Part model, mm, in its own coordinate system. A direction names the side the tool comes from. Coordinates: 2 decimals unless noted, no trailing zeros. Loops run counter-clockwise (first coordinate to the right, second up) from the corner with the lowest first, then second, coordinate; pieces in that order, holes last. Notation, with made-up numbers: (14, 18.5) -> (32, 18.5) arc R19 ccw to (32, 40.5) -> close; hole circle Ø9 at (37.5, 24). An arc over 180 degrees is marked (long way). Use one line per item in the form item = value. Start each with the question number.
(1) 3-axis set-ups, long thin cutter, end or side, ignore diameter. For faces 1 (the flat face through (6.261, -1.821, -8.524)), 2 (the flat face through (6, -2.473, 4)), 3 (the flat face through (6, 2.607, 4)): which of +Z, -Z, +X, -X, +Y, -Y reach the whole face in a straight line?
(2) Band-saw the part on C-C on y = 3.25. Give the cut face in (x, z) (1 decimal), then the cut area to 3 significant figures.
(3) Band-saw the part on D-D on y = -0.75. Give the cut face in (x, z) (1 decimal), then the cut area to 3 significant figures.
(4) Drill centre lines: L1, parallel to Z at x = 8.5, y = -4 (3 decimals); L2, parallel to Y at x = 5, z = 3.75; L3, parallel to Y at x = 10, z = -4. Where is each one in solid material? Low to high. Write a range as [from, to].
(5) Pin check, flat tips, straight feed: P1, Ø3, axis at x = -3, y = 2, coming from the +Z side; P2, Ø0.7, axis at x = -4, z = 4.5, coming from the +Y side; P3, Ø6, axis at x = -7, y = -4.5, coming from the -Z side. Stop position of each tip, or through.
```python
from build123d import *

# Parameters (mm, degrees)
F0_W      = 25.4
F0_H      = 12.7
F3_DEPTH  = 3.175
F3_FACE_W = 25.4
F3_FACE_H = 12.7
F4_DEPTH  = 3.175
F5_W      = 5.08
F5_H      = 2.286
F7_DEPTH  = 12.7
F6_W      = 5.08
F6_H      = 2.286
F8_DEPTH  = 12.7
F9_DEPTH  = 12.7


with BuildPart() as f3:
    # F0 (on Top) → F3 (new body)
    with BuildSketch(Plane.XY):
        Rectangle(F0_W, F0_H)
    extrude(amount=F3_DEPTH)

    # F3_face (on face) → F4 (join)
    with BuildSketch(Plane(origin=(0, 0, 0), x_dir=(1, 0, 0), z_dir=(0, 0, -1))):
        Rectangle(F3_FACE_W, F3_FACE_H)
    extrude(amount=F4_DEPTH)

    # F1 (on Right) + F5 (on Right) → F7 (join)
    with BuildSketch(Plane.YZ):
        Polygon((3.592102, 6.754402), (0, 10.346504), (-3.592102, 6.754402), (0, 3.1623), align=None)
    with BuildSketch(Plane.YZ):
        with Locations((0.06673, 4.330203)):
            Rectangle(F5_W, F5_H)
    extrude(amount=F7_DEPTH)

    # F6 (on Right) + F2 (on Right) → F8 (join)
    with BuildSketch(Plane.YZ):
        with Locations((-0.087894, -4.272406)):
            Rectangle(F6_W, F6_H)
    with BuildSketch(Plane.YZ):
        Polygon((0, -10.345057), (3.592102, -6.752954), (0, -3.160852), (-3.592102, -6.752954), align=None)
    extrude(amount=F8_DEPTH)

    # F7_face (on face) + F8_face (on face) → F9 (join)
    with BuildSketch(Plane(origin=(0, 0.024156, 6.218296), x_dir=(0, 1, 0), z_dir=(-1, 0, 0))):
        Polygon((-0.04906, 3.031093), (-2.497427, 3.031093), (-2.497427, 0.745093), (-2.33506, 0.745093), (-3.616259, -0.536106), (-0.024156, -4.128208), (3.567946, -0.536106), (2.286747, 0.745093), (2.582573, 0.745093), (2.582573, 3.031093), (0.000747, 3.031093), (-0.011456, 3.043296), (-0.036857, 3.043296), align=None)
    with BuildSketch(Plane(origin=(0, -0.031159, -6.212423), x_dir=(0, 1, 0), z_dir=(-1, 0, 0))):
        Polygon((-2.596735, -3.037423), (2.483265, -3.037423), (2.483265, -0.797017), (2.285713, -0.797017), (3.623261, 0.540531), (0.031159, 4.132633), (-3.560944, 0.540531), (-2.223395, -0.797017), (-2.596735, -0.797017), align=None)
    extrude(amount=F9_DEPTH)


solid = f3.part
```
A:
q1.face_1 = -Z, +X, -X, -Y
q1.face_2 = +X, -X, -Y
q1.face_3 = +X, -X, +Y
q2.outline = (-12.7, -7.1) -> (12.7, -7.1) -> (12.7, -6.4) -> (-12.7, -6.4) -> close; (-12.7, -3.2) -> (12.7, -3.2) -> (12.7, 3.2) -> (-12.7, 3.2) -> close; (-12.7, 6.4) -> (12.7, 6.4) -> (12.7, 7.1) -> (-12.7, 7.1) -> close
q2.area = 196 mm²
q3.outline = (-12.7, -9.6) -> (12.7, -9.6) -> (12.7, 3.2) -> (-12.7, 3.2) -> close; (-12.7, 3.2) -> (12.7, 3.2) -> (12.7, 9.6) -> (-12.7, 9.6) -> close
q3.area = 487 mm²
q4.L1 = [-3.175, 3.175]
q4.L2 = [-2.47, 2.61]
q4.L3 = [-2.63, 2.45]
q5.P1 = 9.85
q5.P2 = 2.61
q5.P3 = -8.85
